Can you work these out from the drawing? Everything is in mm from the part's minimum corner. Coordinates: 2 decimals unless noted, no trailing zeros. Order: outer loops, then holes, each group sorted by start corner. A loop starts at its lowest first (then second) coordinate and runs counter-clockwise, first axis right, second up. Notation, with made-up numbers: (86.5, 67.25) -> (109.5, 67.25) arc R20 ccw to (109.5, 76.25) -> close; hole circle Ø7 at (34, 74.5). An arc over 180 degrees is marked (long way). Use a Markdown table: item, result. Add a question column.
1) If we section it at B-B (z = 21.5): Write out the boundary of the cut face in (x, y), plus the area to 3 significant figures.
2) If I drill on L1, parallel to X at y = 9, z = 9; L2, parallel to Z at x = 16, y = 11; L3, parallel to Y at x = 24, z = 6, over which ranges is the centre line in solid material (lowest first)? Write a range as [from, to].
3) If we section it at D-D (z = 6): Write out the boundary of the cut face in (x, y).
4) If we section it at A-A (x = 20.25): Write out the boundary of the cut face in (y, z), plus the area to 3 significant figures.
5) If we section it at C-C (y = 38): Write out the boundary of the cut face in (x, z), plus the area to 3 significant figures.
6) Will these pins go through, and if not, where does the flat tip stop? pin 1 Ø8 at (x, z) = (11.5, 12) entering from +Y (1 decimal); pin 2 Ø10 at (x, z) = (6, 11.5) entering from +Y (1 decimal); pin 3 Ø10 at (x, y) = (13, 36.5) entering from +Z; pin 4 Ø12 at (x, y) = (10, 6) entering from -Z.
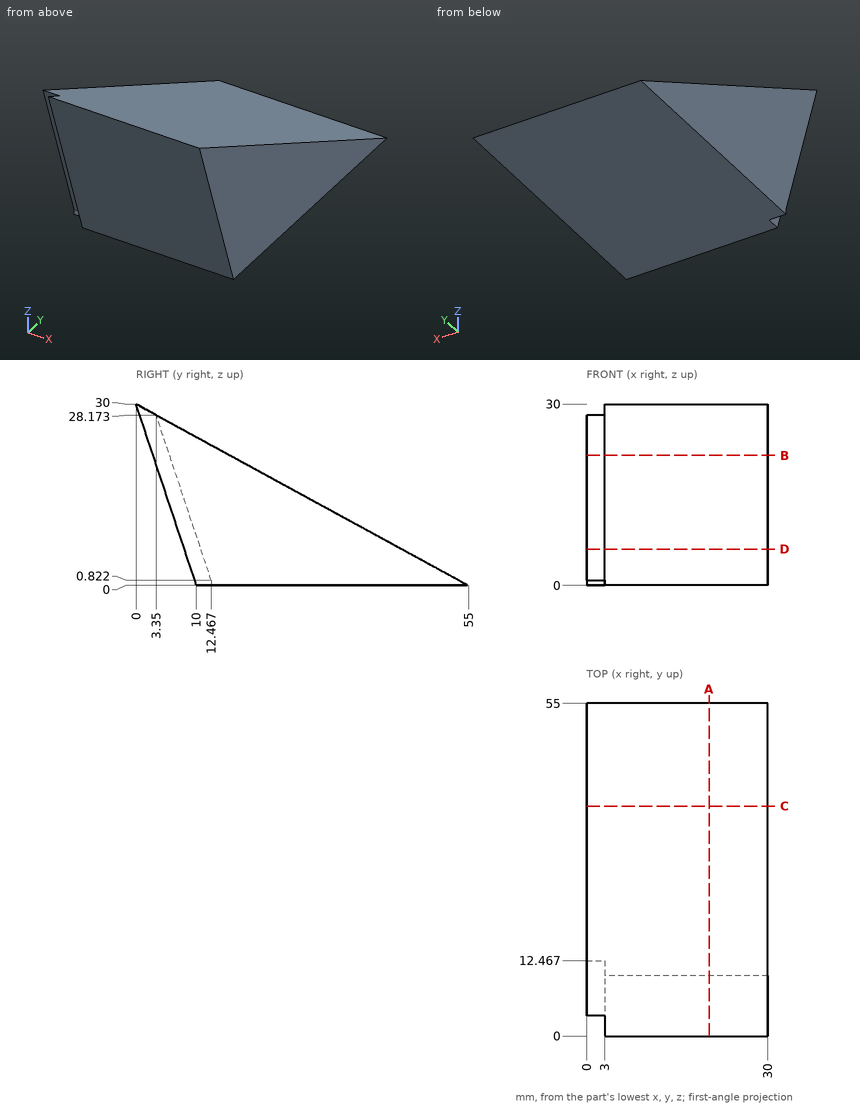
Answer sheet:
| question | item | result |
|---|---|---|
| 1 | outline | (0, 5.57) -> (3, 5.57) -> (3, 2.83) -> (30, 2.83) -> (30, 15.58) -> (0, 15.58) -> close |
| 1 | area | 374 mm2 |
| 2 | L1 | [3, 30] |
| 2 | L2 | [0, 24] |
| 2 | L3 | [8, 44] |
| 3 | outline | (0, 10.74) -> (3, 10.74) -> (3, 8) -> (30, 8) -> (30, 44) -> (0, 44) -> close |
| 4 | outline | (0, 30) -> (10, 0) -> (55, 0) -> close |
| 4 | area | 675 mm2 |
| 5 | outline | (0, 0) -> (30, 0) -> (30, 9.27) -> (0, 9.27) -> close |
| 5 | area | 278 mm2 |
| 6 | pin 1 | y = 40.3 |
| 6 | pin 2 | y = 43.1 |
| 6 | pin 3 | z = 12.82 |
| 6 | pin 4 | z = 0 |
